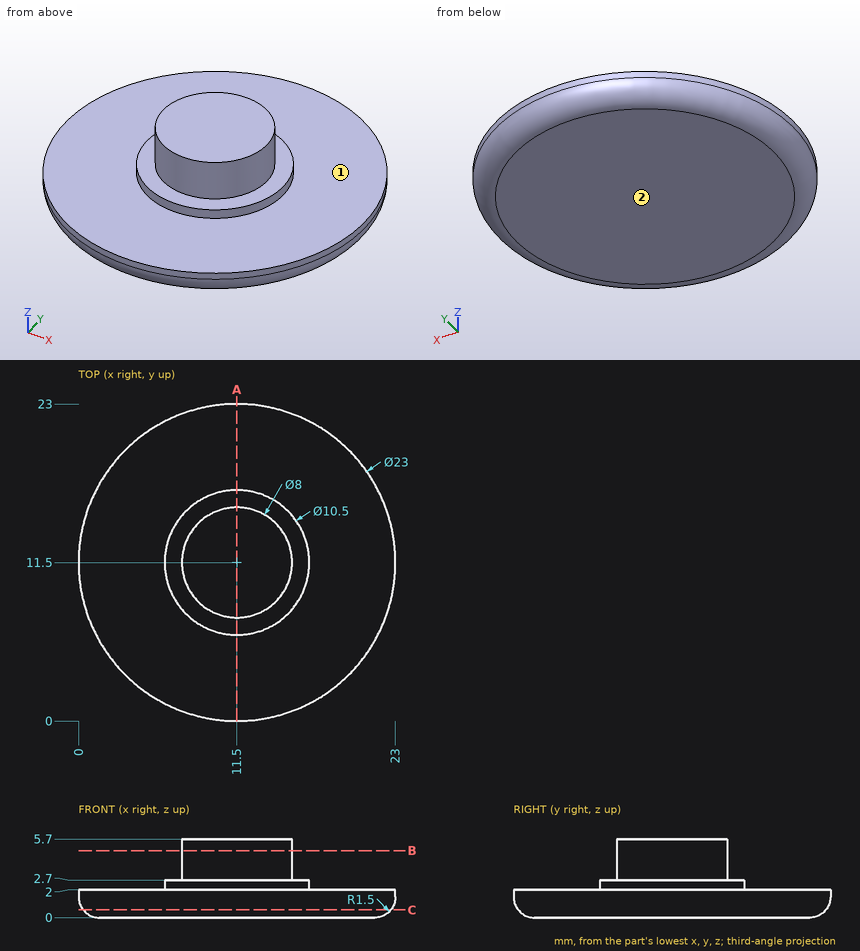
The drawing under review shows one solid part. Ordinate dimensions are in mm from its lowest x, y, z. A direction names the side the tool comes from. Give positions to 0.01 mm unless a question says otherwise; leave off trailing zeros. Write each loop counter-clockwise with the first axis right and the second up, starting at its lowest first coordinate (ties: lowest second). Pieces come first, ordered by that corner, then holes. Notation, with made-up numbers: M 17.5,72.25 L 29.5,72.25 A16 cw 29.5,88.25 Z; hole C 33.25,-39 d4. An arc over 180 degrees is marked long. Write each question's results on one line, items separated by ' | '. Start each with the question number.
1. Insertion check: pin 1 Ø2 at (x, y) = (12, 20) entering from +Z; pin 2 Ø1 at (x, z) = (5, 1) entering from +Y; pin 3 Ø3 at (x, z) = (18, 1.5) entering from -Y. Each pin has a flat end and moves straight along its axis. Give the tip position at first contact, or say it passes through.
2. We need section C-C (z = 0.55). Write out the cut boundary in (x, y), and give its area (3 significant figures).
3. We need section A-A (x = 11.5). Write out the cut boundary in (y, z), and give its area (3 significant figures).
4. For probe 1 along Z at (x, y) = (7.5, 7.5); probe 2 along Y at (x, z) = (8.25, 4.75); probe 3 along X at (y, z) = (12.5, 2.1), list the stretches that pass through material, from the lowest coordinate up. Write a range as [from, to].
5. We need section B-B (z = 4.85). Write out the cut boundary in (x, y), and give its area (3 significant figures).
6. For the marked faces 1 and 2, list the 3-axis set-ups (+Z, -Z, +X, -X, +Y, -Y) from which the entire face can be reached by the end or side of a thin tool; tool diameter is ignored.
Results found:
1) pin 1: stops at z = 2 | pin 2: stops at y = 21.25 | pin 3: stops at y = 1.14
2) outline: C 11.5,11.5 d22.32 | area: 391 mm^2
3) outline: M 0,1.5 A1.5 ccw 1.5,0 L 21.5,0 A1.5 ccw 23,1.5 L 23,2 L 16.75,2 L 16.75,2.7 L 15.5,2.7 L 15.5,5.7 L 7.5,5.7 L 7.5,2.7 L 6.25,2.7 L 6.25,2 L 0,2 Z | area: 76.4 mm^2
4) probe 1: z = [0, 2] | probe 2: y = [9.17, 13.83] | probe 3: x = [6.35, 16.65]
5) outline: C 11.5,11.5 d8 | area: 50.3 mm^2
6) face 1: +Z | face 2: -Z, +X, -X, +Y, -Y
